from build123d import *

# Parameters (mm, degrees)
SKETCH1_W           = 20
SKETCH1_H           = 23
SKETCH1_W_2         = 8
SKETCH1_H_2         = 11
BOSS_EXTRUDE1_DEPTH = 8
CHAMFER1_SIZE       = 1.5
CHAMFER2_SIZE       = 0.6


with BuildPart() as part:
    # Sketch1 → Boss-Extrude1 (new body)
    with BuildSketch(Plane(origin=(0, 0, 0), x_dir=(1, 0, 0), z_dir=(0, 1, 0))):
        Rectangle(SKETCH1_W, SKETCH1_H)
        Rectangle(SKETCH1_W_2, SKETCH1_H_2, mode=Mode.SUBTRACT)
    extrude(amount=BOSS_EXTRUDE1_DEPTH)

    # Chamfer1
    chamfer1_edges = [part.edges().sort_by_distance(p)[0] for p in [
        (-10, 4, -11.5),
        (10, 4, -11.5),
        (10, 4, 11.5),
        (-10, 4, 11.5),
    ]]
    chamfer(chamfer1_edges, length=CHAMFER1_SIZE)

    # Chamfer2
    chamfer2_edges = [part.edges().sort_by_distance(p)[0] for p in [
        (10, 8, 0),
        (0, 8, 11.5),
        (-10, 8, 0),
        (0, 8, -11.5),
        (-9.25, 8, 10.75),
        (9.25, 8, -10.75),
        (9.25, 8, 10.75),
    ]]
    chamfer(chamfer2_edges, length=CHAMFER2_SIZE)


solid = part.part
Geometry: final body of the model. Coordinates: model frame, mm. A direction names the side the tool comes from. Coordinates: 2 decimals unless noted, no trailing zeros. Write each loop counter-clockwise with the first axis right and the second up, starting at its lowest first coordinate (ties: lowest second). Pieces come first, ordered by that corner, then holes. Notation, with made-up numbers: (7.5, -14) - (18.5, -14) arc R28 cw to (18.5, 12) - close; hole circle Ø4 at (-27.75, 36.25). An arc over 180 degrees is marked (long way). Return JSON: item names as keys, results as strings.
Item 1: Section query A-A (z = -4.75). Output: boundary loops of the cut face in (x, y).
Completed:
{"outline": "(-10, 0) - (-4, 0) - (-4, 8) - (-9.4, 8) - (-10, 7.4) - close; (4, 0) - (10, 0) - (10, 7.4) - (9.4, 8) - (4, 8) - close"}
Item 2: Line query: L1, parallel to Z at x = -1.75, y = 5.5; L2, parallel to X at y = 3.75, z = 1.5; L3, parallel to Z at x = -7.5, y = 7.75. Output: solid intervals per line, ascending.
Completed:
{"L1": "z = -11.5 to -5.5, 5.5 to 11.5", "L2": "x = -10 to -4, 4 to 10", "L3": "z = -11.15 to 11.15"}
Item 3: Pin query (flat end, axial travel): pin 1 Ø5 at (x, z) = (3.5, 2) entering from -Y. Return the tip coordinate at first contact, or that it passes through.
Completed:
{"pin 1": "stops at y = 0"}
Item 4: Pull-direction query (Z, two-part tool) for faces 1 (the face through (9.03, 7.696, -10.551)), 2 (the face through (0, 4, -5.5)), 3 (the face through (9, 4, 11)), 4 (the face through (-4, 4, 0)); classes: +Z half, -Z half, draft (parallel to the pull), parting line (faces both ways), or undercut.
Completed:
{"face 1": "-Z half", "face 2": "undercut", "face 3": "+Z half", "face 4": "undercut"}
Item 5: Section query B-B (x = 3.5). Output: boundary loops of the cut face in (y, z), and give its area (3 significant figures).
Completed:
{"outline": "(0, -11.5) - (7.4, -11.5) - (8, -10.9) - (8, -5.5) - (0, -5.5) - close; (0, 5.5) - (8, 5.5) - (8, 10.9) - (7.4, 11.5) - (0, 11.5) - close", "area": "95.6 mm2"}
Item 6: Reachability of faces 5 (the face through (0, 4, 5.5)), 6 (the face through (0, 4, 11.5)) from +Z, -Z, +X, -X, +Y, -Y: full face, straight path, thin tool, end or side. Return the list, or none.
Completed:
{"face 5": "+Y, -Y", "face 6": "+Z, +X, -X, +Y, -Y"}
Item 7: Section query C-C (y = 4.5). Output: boundary loops of the cut face in (x, z), and give its area (4 significant figures).
Completed:
{"outline": "(-10, -10) - (-8.5, -11.5) - (8.5, -11.5) - (10, -10) - (10, 10) - (8.5, 11.5) - (-8.5, 11.5) - (-10, 10) - close; hole (-4, -5.5) - (4, -5.5) - (4, 5.5) - (-4, 5.5) - close", "area": "367.5 mm2"}
